Design review of the part built by this model. Coordinates are the model's own, in mm. Round coordinates to 2 decimals unless told otherwise and drop trailing zeros. Order: outer loops, then holes, each group sorted by start corner. A loop starts at its lowest first (then second) coordinate and runs counter-clockwise, first axis right, second up. Notation, with made-up numbers: (-5.75, -17.75) - (2.25, -17.75) arc R24 cw to (2.25, 1.25) - close; hole circle Ø5 at (77, -20). An arc over 180 degrees is marked (long way). Write item = value, one per line.
from build123d import *

# Parameters (mm, degrees)
SKETCH1_W            = 40
SKETCH1_H            = 40
BOSS_EXTRUDE1_DEPTH  = 2
SKETCH2_R            = 1.65
CUT_EXTRUDE1_DEPTH   = 3
LPATTERN1_COUNT      = 4
LPATTERN1_PITCH      = 10
LPATTERN1_COUNT_DIR2 = 4
LPATTERN1_PITCH_DIR2 = 10


with BuildPart() as part:
    # Sketch1 → Boss-Extrude1 (new body)
    with BuildSketch(Plane.XY):
        Rectangle(SKETCH1_W, SKETCH1_H)
    extrude(amount=BOSS_EXTRUDE1_DEPTH)

    # Sketch2 → Cut-Extrude1 (cut, through all)
    with BuildSketch(Plane.XY.offset(2)):
        with Locations((-15, 15)):
            Circle(SKETCH2_R)
    cut_extrude1 = extrude(amount=-CUT_EXTRUDE1_DEPTH, mode=Mode.SUBTRACT)

    # LPattern1: Cut-Extrude1 4 × 4
    with Locations(*[(j * LPATTERN1_PITCH_DIR2, -i * LPATTERN1_PITCH, 0) for i in range(LPATTERN1_COUNT) for j in range(LPATTERN1_COUNT_DIR2) if (i, j) != (0, 0)]):
        add(cut_extrude1, mode=Mode.SUBTRACT)


solid = part.part
Item 1: Take a section at A-A, the plane x = -5. State the section outline as (y, z) points.
Data:
outline = (-20, 0) - (-16.65, 0) - (-16.65, 2) - (-20, 2) - close; (-13.35, 0) - (-6.65, 0) - (-6.65, 2) - (-13.35, 2) - close; (-3.35, 0) - (3.35, 0) - (3.35, 2) - (-3.35, 2) - close; (6.65, 0) - (13.35, 0) - (13.35, 2) - (6.65, 2) - close; (16.65, 0) - (20, 0) - (20, 2) - (16.65, 2) - close
Item 2: The part is to be moulded in two halves that separate along Y. For faces 1 (the face through (-6.216, -13.885, 1.014)), 2 (the face through (0, 0, 0)), 3 (the face through (3.784, -13.885, 1.014)), 4 (the face through (0, -20, 1)), say which applies: +Y half, -Y half, draft (parallel to the pull), parting line (faces both ways), or undercut.
Data:
face_1 = undercut
face_2 = draft
face_3 = undercut
face_4 = -Y half
Item 3: Insertion check: P1, Ø2, axis at x = -5, y = -15, coming from the +Z side. The pin has a flat end and moves straight along its axis. Give the tip position at first contact, or say it passes through.
Data:
P1 = through
Item 4: Take a section at C-C, the plane z = 1.4. Count the separate pieces of the cut face and the enclosed holes in it, and give its area (3 significant figures).
Data:
separate_pieces = 1
enclosed_holes = 16
area = 1,460 mm2
Item 5: For line 1 along Y through (x, z) = (-15, 1.1); line 2 along Y through (x, z) = (3.5, 1.7); line 3 along X through (y, z) = (15.5, 1.5), list the stretches that pass through material, from the lowest coordinate up. Write a range as [from, to].
Data:
line_1 = [-20, -16.65], [-13.35, -6.65], [-3.35, 3.35], [6.65, 13.35], [16.65, 20]
line_2 = [-20, -15.69], [-14.31, -5.69], [-4.31, 4.31], [5.69, 14.31], [15.69, 20]
line_3 = [-20, -16.57], [-13.43, -6.57], [-3.43, 3.43], [6.57, 13.43], [16.57, 20]
